from build123d import *

# Parameters (mm, degrees)
EXTRUDE_1_DEPTH          = 50
CUT_EXTRUDE_1_DEPTH      = 87
CUT_EXTRUDE_1_DEPTH_BACK = 1
SKETCH_3_R               = 2
CUT_EXTRUDE_2_DEPTH      = 20


with BuildPart() as part:
    # Эскиз1 → Бобышка-Вытянуть1 (new body)
    with BuildSketch(Plane.XY):
        with BuildLine():
            Line((0, 20), (0, 0))
            ThreePointArc((0, 0), (43, -43), (86, 0))
            Line((86, 0), (86, 20))
            Line((86, 20), (0, 20))
        make_face()
    extrude(amount=EXTRUDE_1_DEPTH)

    # Эскиз2 → Вырез-Вытянуть1 (cut, two sides)
    with BuildSketch(Plane(origin=(0, 0, 0), x_dir=(0, 0, -1), z_dir=(1, 0, 0))) as cut_extrude_1_sk:
        Polygon((-40, 20), (0, -28), (0, 20), align=None)
    extrude(amount=CUT_EXTRUDE_1_DEPTH, mode=Mode.SUBTRACT)
    extrude(cut_extrude_1_sk.sketch, amount=-CUT_EXTRUDE_1_DEPTH_BACK, mode=Mode.SUBTRACT)

    # Эскиз3 → Вырез-Вытянуть2 (cut)
    with BuildSketch(Plane(origin=(0, -43, 0), x_dir=(-1, 0, 0), z_dir=(0, -1, 0))):
        with Locations((-43, -38)):
            Circle(SKETCH_3_R)
    extrude(amount=-CUT_EXTRUDE_2_DEPTH, mode=Mode.SUBTRACT)


solid = part.part
Design review of the part built by this model. Coordinates are the model's own, in mm. A direction names the side the tool comes from. Round coordinates to 2 decimals unless told otherwise and drop trailing zeros. Loops run counter-clockwise (first coordinate to the right, second up) from the corner with the lowest first, then second, coordinate; pieces in that order, holes last. Notation, with made-up numbers: M -34.5,-3 L -11.5,-3 A23 cw -11.5,20 Z; hole C 52,3 d10. An arc over 180 degrees is marked long. Answer as a JSON object with one key per item and string values.
Item 1: We need section C-C on z = 43. Give the boundary of the cut face in (x, y), and give its area (3 significant figures).
Answer sheet:
{"outline": "M 0,0 A43 ccw 86,0 L 86,20 L 0,20 Z", "area": "4,620 mm^2"}
Item 2: We need section B-B on y = -24. Give the boundary of the cut face in (x, z), and give its area (3 significant figures).
Answer sheet:
{"outline": "M 7.32,3.33 L 78.68,3.33 L 78.68,50 L 7.32,50 Z; hole C 43,38 d4", "area": "3,320 mm^2"}
Item 3: We need section A-A on x = 43. Give the boundary of the cut face in (y, z).
Answer sheet:
{"outline": "M -43,0 L -28,0 L 20,40 L 20,50 L -43,50 L -43,40 L -23,40 L -23,36 L -43,36 Z"}
Item 4: The part is to be moulded in two halves that separate along X. For faces 1 (the flat face through (44, 20, 45)), 2 (the cylindrical face through (42.05, -42.99, 24.65)), 3 (the cylindrical face through (43, -33, 40)), say which applies: pulls with the +X half, pulls with the -X half, needs draft (parallel to the pull), parting line crosses it, or undercut.
Answer sheet:
{"face 1": "needs draft", "face 2": "parting line crosses it", "face 3": "undercut"}
Item 5: Clearance check with flat-ended pins moving along their axes: P1, Ø2, axis at y = -21.5, z = 16.5, coming from the -X side; P2, Ø1.5, axis at x = 60, z = 33, coming from the -Y side; P3, Ø3, axis at x = 56, z = 30.5, coming from the -Y side. State where each tip first meets the part, or that it passes through.
Answer sheet:
{"P1": "stops at x = 5.2", "P2": "stops at y = -39.81", "P3": "stops at y = -41.43"}
Item 6: Machinability: for faces 4 (the flat face through (42, -4, 50)), 5 (the flat face through (43, -23, 38)), which of the approach directions +Z, -Z, +X, -X, +Y, -Y give a long, thin tool a straight path to every point of the face, cutting with its end or side? Answer none if there is none.
Answer sheet:
{"face 4": "+Z, +X, -X, +Y, -Y", "face 5": "-Y"}
Item 7: We need section D-D on y = 15.5. Give the boundary of the cut face in (x, z), and give its area (3 significant figures).
Answer sheet:
{"outline": "M 0,36.25 L 86,36.25 L 86,50 L 0,50 Z", "area": "1,180 mm^2"}
Item 8: Wall thickness on L1, parallel to Z at x = 43, y = -35.75; L2, parallel to X at y = -33, z = 38; L3, parallel to X at y = -27.5, z = 38: over which ranges is each line inside the solid? List them lowest first. Write a range as from..to.
Answer sheet:
{"L1": "z = 0..36, 40..50", "L2": "x = 15.43..41, 45..70.57", "L3": "x = 9.94..41, 45..76.06"}
